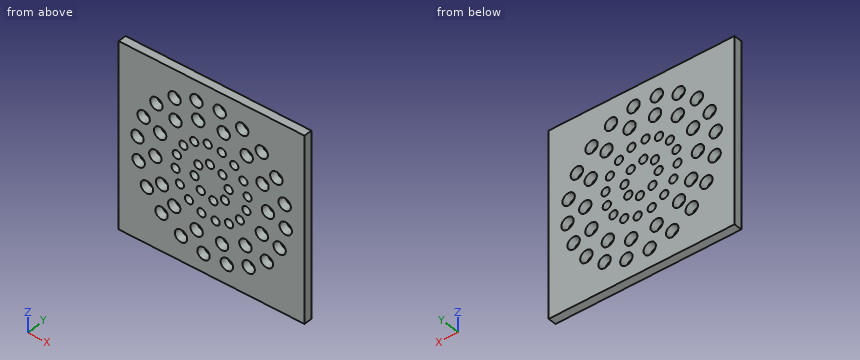
from build123d import *

# Parameters (mm, degrees)
F0_W     = 45
F0_H     = 45
F1_DEPTH = 2
F2_R     = 1
F2_R_2   = 1.5
F3_DEPTH = 19.6
F4_DEPTH = 25


# Not quite as in the source:
# - a feature names something its author has since deleted; it is built from what else it names


with BuildPart() as f1:
    # F0 (on Front) → F1 (new body)
    with BuildSketch(Plane.XZ):
        with Locations((-22.5, 22.5)):
            Rectangle(F0_W, F0_H)
    extrude(amount=F1_DEPTH)

    # F2 (on face) → F3 (cut)
    with BuildSketch(Plane.XZ.offset(2)):
        with Locations((-26.6271115437, 22.0804515862)):
            Circle(F2_R)
        with Locations((-25.7149740877, 25.1216430309)):
            Circle(F2_R)
        with Locations((-22.9195484138, 26.6271115437)):
            Circle(F2_R)
        with Locations((-25.1216430309, 19.2850259123)):
            Circle(F2_R)
        with Locations((-10.3415464992, 16.307327403)):
            Circle(F2_R_2)
        with Locations((-8.8567808269, 22.3006108876)):
            Circle(F2_R_2)
        with Locations((-10.1657718628, 28.3347237882)):
            Circle(F2_R_2)
        with Locations((-14.0004741816, 33.1740454509)):
            Circle(F2_R_2)
        with Locations((-34.5032584426, 16.011627925)):
            Circle(F2_R_2)
        with Locations((-40.4566549108, 24.4574602037)):
            Circle(F2_R_2)
        with Locations((-40.1826821325, 18.8127437526)):
            Circle(F2_R_2)
        with Locations((-29.9105668117, 6.027094805)):
            Circle(F2_R_2)
        with Locations((-19.5756460311, 35.8276156641)):
            Circle(F2_R_2)
        with Locations((-18.8127437526, 4.8173178675)):
            Circle(F2_R_2)
        with Locations((-38.1778052247, 13.5289616335)):
            Circle(F2_R_2)
        with Locations((-34.6382755077, 9.1233272547)):
            Circle(F2_R_2)
        with Locations((-24.4574602037, 4.5433450892)):
            Circle(F2_R_2)
        with Locations((-25.7496452846, 35.7520561027)):
            Circle(F2_R_2)
        with Locations((-31.2582064036, 32.9628392904)):
            Circle(F2_R_2)
        with Locations((-38.972905195, 29.9105668117)):
            Circle(F2_R_2)
        with Locations((-36.1342532423, 21.9667796436)):
            Circle(F2_R_2)
        with Locations((-34.9733273102, 28.0311202515)):
            Circle(F2_R_2)
        with Locations((-13.5289616335, 6.8221947753)):
            Circle(F2_R_2)
        with Locations((-26.1872562474, 40.1826821325)):
            Circle(F2_R_2)
        with Locations((-31.4710383665, 38.1778052247)):
            Circle(F2_R_2)
        with Locations((-35.8766727453, 34.6382755077)):
            Circle(F2_R_2)
        with Locations((-9.1233272547, 10.3617244923)):
            Circle(F2_R_2)
        with Locations((-6.027094805, 15.0894331883)):
            Circle(F2_R_2)
        with Locations((-4.5433450892, 20.5425397963)):
            Circle(F2_R_2)
        with Locations((-4.8173178675, 26.1872562474)):
            Circle(F2_R_2)
    extrude(amount=-F3_DEPTH, mode=Mode.SUBTRACT)

    # F2 (on face) → F4 (cut)
    with BuildSketch(Plane.XZ.offset(2)):
        with Locations((-22.9195484138, 26.6271115437)):
            Circle(F2_R)
        with Locations((-25.7149740877, 25.1216430309)):
            Circle(F2_R)
        with Locations((-26.6271115437, 22.0804515862)):
            Circle(F2_R)
        with Locations((-25.1216430309, 19.2850259123)):
            Circle(F2_R)
        with Locations((-34.5032584426, 16.011627925)):
            Circle(F2_R_2)
        with Locations((-36.1342532423, 21.9667796436)):
            Circle(F2_R_2)
        with Locations((-34.9733273102, 28.0311202515)):
            Circle(F2_R_2)
        with Locations((-31.2582064036, 32.9628392904)):
            Circle(F2_R_2)
        with Locations((-25.7496452846, 35.7520561027)):
            Circle(F2_R_2)
        with Locations((-19.5756460311, 35.8276156641)):
            Circle(F2_R_2)
        with Locations((-14.0004741816, 33.1740454509)):
            Circle(F2_R_2)
        with Locations((-10.1657718628, 28.3347237882)):
            Circle(F2_R_2)
        with Locations((-8.8567808269, 22.3006108876)):
            Circle(F2_R_2)
        with Locations((-10.3415464992, 16.307327403)):
            Circle(F2_R_2)
        with Locations((-26.1872562474, 40.1826821325)):
            Circle(F2_R_2)
        with Locations((-31.4710383665, 38.1778052247)):
            Circle(F2_R_2)
        with Locations((-35.8766727453, 34.6382755077)):
            Circle(F2_R_2)
        with Locations((-38.972905195, 29.9105668117)):
            Circle(F2_R_2)
        with Locations((-40.4566549108, 24.4574602037)):
            Circle(F2_R_2)
        with Locations((-40.1826821325, 18.8127437526)):
            Circle(F2_R_2)
        with Locations((-38.1778052247, 13.5289616335)):
            Circle(F2_R_2)
        with Locations((-34.6382755077, 9.1233272547)):
            Circle(F2_R_2)
        with Locations((-29.9105668117, 6.027094805)):
            Circle(F2_R_2)
        with Locations((-24.4574602037, 4.5433450892)):
            Circle(F2_R_2)
        with Locations((-18.8127437526, 4.8173178675)):
            Circle(F2_R_2)
        with Locations((-13.5289616335, 6.8221947753)):
            Circle(F2_R_2)
        with Locations((-9.1233272547, 10.3617244923)):
            Circle(F2_R_2)
        with Locations((-6.027094805, 15.0894331883)):
            Circle(F2_R_2)
        with Locations((-4.5433450892, 20.5425397963)):
            Circle(F2_R_2)
        with Locations((-4.8173178675, 26.1872562474)):
            Circle(F2_R_2)
        with Locations((-14.3160296348, 11.5821332447)):
            Circle(F2_R_2)
        with Locations((-19.966365208, 9.0926184449)):
            Circle(F2_R_2)
        with Locations((-26.1355196249, 9.3485672841)):
            Circle(F2_R_2)
        with Locations((-31.5602194369, 12.2975684673)):
            Circle(F2_R_2)
        with Locations((-6.8221947753, 31.4710383665)):
            Circle(F2_R_2)
        with Locations((-10.3617244923, 35.8766727453)):
            Circle(F2_R_2)
        with Locations((-15.0894331883, 38.972905195)):
            Circle(F2_R_2)
        with Locations((-20.5425397963, 40.4566549108)):
            Circle(F2_R_2)
        with Locations((-26.7185367273, 30.1892252677)):
            Circle(F2_R)
        with Locations((-29.3399588572, 27.9895537314)):
            Circle(F2_R)
        with Locations((-30.9200592554, 24.9541474023)):
            Circle(F2_R)
        with Locations((-31.2182819601, 21.5451193782)):
            Circle(F2_R)
        with Locations((-30.1892252677, 18.2814632727)):
            Circle(F2_R)
        with Locations((-27.9895537314, 15.6600411428)):
            Circle(F2_R)
        with Locations((-24.9541474023, 14.0799407446)):
            Circle(F2_R)
        with Locations((-21.5451193782, 13.7817180399)):
            Circle(F2_R)
        with Locations((-18.2814632727, 14.8107747323)):
            Circle(F2_R)
        with Locations((-15.6600411428, 17.0104462686)):
            Circle(F2_R)
        with Locations((-22.0804515862, 18.3728884563)):
            Circle(F2_R)
        with Locations((-19.2850259123, 19.8783569691)):
            Circle(F2_R)
        with Locations((-18.3728884563, 22.9195484138)):
            Circle(F2_R)
        with Locations((-19.8783569691, 25.7149740877)):
            Circle(F2_R)
        with Locations((-14.0799407446, 20.0458525977)):
            Circle(F2_R)
        with Locations((-13.7817180399, 23.4548806218)):
            Circle(F2_R)
        with Locations((-14.8107747323, 26.7185367273)):
            Circle(F2_R)
        with Locations((-17.0104462686, 29.3399588572)):
            Circle(F2_R)
        with Locations((-20.0458525977, 30.9200592554)):
            Circle(F2_R)
        with Locations((-23.4548806218, 31.2182819601)):
            Circle(F2_R)
    extrude(amount=-F4_DEPTH, mode=Mode.SUBTRACT)


solid = f1.part
Build history of the part. All positions in model axes, mm. Give positions to 0.01 mm unless a question says otherwise; leave off trailing zeros. Order: outer loops, then holes, each group sorted by start corner. A loop starts at its lowest first (then second) coordinate and runs counter-clockwise, first axis right, second up. Notation, with made-up numbers: M 24,9.5 L 63,9.5 A16 ccw 63,26.5 Z; hole C 73,-34 d7. An arc over 180 degrees is marked long. Put each result on its own line as item: value.
Item 1: Drop flat-ended pins along their axis: pin 1 Ø1.6 at (x, z) = (-14.08, 20.05) entering from -Y; pin 2 Ø2.5 at (x, z) = (-24.95, 14.08) entering from +Y. Give the stop position or say it passes through.
Results are:
pin 1: through
pin 2: y = 0
Item 2: Cut at B-B on y = -0.45. Count the separate pieces of the cut face and the enclosed holes in it, then the cut area to 3 significant figures.
Results are:
separate pieces: 1
enclosed holes: 58
area: 1,710 mm2
Item 3: Wall check: probe 1 along X at (y, z) = (-0.85, 11); probe 2 along X at (y, z) = (-1.65, 17); probe 3 along X at (y, z) = (-0.45, 15.5). Give the ranges that are in metal, low to high.
Results are:
probe 1: -45 to -32.31, -30.81 to -15.7, -12.93 to -10.48, -7.77 to 0
probe 2: -45 to -35.63, -33.37 to -16.66, -14.66 to -11.67, -9.01 to 0
probe 3: -45 to -35.91, -33.09 to -28.98, -27 to -19.01, -17.56 to -11.61, -9.08 to -7.47, -4.58 to 0
Item 4: Cut at A-A on z = 4. Write the cut outline in (x, y), then the cut area to 3 significant figures.
Results are:
outline: M -45,-2 L -25.86,-2 L -25.86,0 L -45,0 Z; M -23.06,-2 L -20.07,-2 L -20.07,0 L -23.06,0 Z; M -17.55,-2 L 0,-2 L 0,0 L -17.55,0 Z
area: 79.4 mm2
